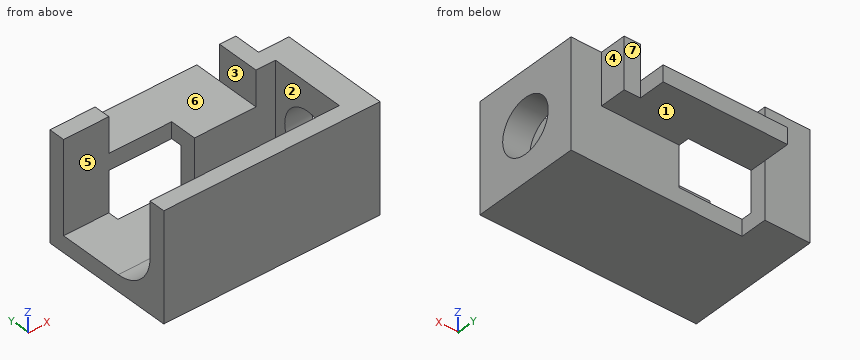
from build123d import *

# Parameters (mm, degrees)
F0_W      = 40
F0_H      = 20
F1_DEPTH  = 10
F3_W      = 35
F3_H      = 3
F4_DEPTH  = 10
F5_W      = 23
F5_H      = 3
F6_DEPTH  = 6.5
F7_W      = 23
F7_H      = 3
F8_DEPTH  = 5
F9_DEPTH  = 10
F10_DEPTH = 35
F11_DEPTH = 40
F12_DEPTH = 35
F13_DEPTH = 40
F14_DEPTH = 35
F15_W     = 20
F15_H     = 17
F16_DEPTH = 5


with BuildPart() as f1:
    # F0 (on Top) → F1 (new body)
    with BuildSketch(Plane.XY):
        Rectangle(F0_W, F0_H)
    extrude(amount=F1_DEPTH)

    # F3 (on face) → F4 (join)
    with BuildSketch(Plane.XY.offset(10)):
        Polygon((20, -10), (20, 10), (15, 10), (15, 7), (15, -7), (15, -10), align=None)
        with Locations((-2.5, 8.5)):
            Rectangle(F3_W, F3_H)
        with Locations((-2.5, -8.5)):
            Rectangle(F3_W, F3_H)
    extrude(amount=F4_DEPTH)

    # F5 (on face) → F6 (cut)
    with BuildSketch(Plane.XY.offset(20)):
        with Locations((-0.1296941414, 8.5)):
            Rectangle(F5_W, F5_H)
    extrude(amount=-F6_DEPTH, mode=Mode.SUBTRACT)

    # F7 (on face) → F8 (join)
    with BuildSketch(Plane(origin=(0, 10, 0), x_dir=(-1, 0, 0), z_dir=(0, 1, 0))):
        with Locations((0.1296941414, 12)):
            Rectangle(F7_W, F7_H)
        Polygon((-11.3703058586, 10.5), (-11.3703058586, 13.5), (-11.3703058586, 20), (-14.3703058586, 20), (-14.3703058586, 10.5), align=None)
        Polygon((11.6296941414, 20), (11.6296941414, 13.5), (11.6296941414, 10.5), (11.6296941414, 0), (20, 0), (20, 20), align=None)
    extrude(amount=F8_DEPTH)

    # F7 (on face) → F9 (join)
    with BuildSketch(Plane(origin=(0, 10, 0), x_dir=(-1, 0, 0), z_dir=(0, 1, 0))):
        with Locations((0.1296941414, 12)):
            Rectangle(F7_W, F7_H)
    extrude(amount=F9_DEPTH)

    # F2 (on face) → F10 (cut)
    with BuildSketch(Plane(origin=(-20, 0, 0), x_dir=(0, -1, 0), z_dir=(-1, 0, 0))):
        with BuildLine():
            Line((-5, 10), (-7, 10))
            ThreePointArc((-7, 10), (-4.9497474683, 5.0502525317), (0, 3))
            Line((0, 3), (0, 5))
            ThreePointArc((0, 5), (-3.5355339059, 6.4644660941), (-5, 10))
        make_face()
        with BuildLine():
            ThreePointArc((0, 5), (3.5355339059, 6.4644660941), (5, 10))
            Line((5, 10), (0, 10))
            Line((0, 10), (0, 5))
        make_face()
    extrude(amount=-F10_DEPTH, mode=Mode.SUBTRACT)

    # F2 (on face) → F11 (cut)
    with BuildSketch(Plane(origin=(-20, 0, 0), x_dir=(0, -1, 0), z_dir=(-1, 0, 0))):
        with BuildLine():
            Line((0, 10), (5, 10))
            ThreePointArc((5, 10), (0, 15), (-5, 10))
            Line((-5, 10), (0, 10))
        make_face()
        with BuildLine():
            ThreePointArc((0, 5), (3.5355339059, 6.4644660941), (5, 10))
            Line((5, 10), (0, 10))
            Line((0, 10), (0, 5))
        make_face()
        with BuildLine():
            Line((0, 10), (-5, 10))
            ThreePointArc((-5, 10), (-3.5355339059, 6.4644660941), (0, 5))
            Line((0, 5), (0, 10))
        make_face()
    extrude(amount=-F11_DEPTH, mode=Mode.SUBTRACT)

    # F2 (on face) → F12 (cut)
    with BuildSketch(Plane(origin=(-20, 0, 0), x_dir=(0, -1, 0), z_dir=(-1, 0, 0))):
        with BuildLine():
            Line((0, 10), (-5, 10))
            ThreePointArc((-5, 10), (-3.5355339059, 6.4644660941), (0, 5))
            Line((0, 5), (0, 10))
        make_face()
        with BuildLine():
            Line((-5, 10), (-7, 10))
            ThreePointArc((-7, 10), (-4.9497474683, 5.0502525317), (0, 3))
            Line((0, 3), (0, 5))
            ThreePointArc((0, 5), (-3.5355339059, 6.4644660941), (-5, 10))
        make_face()
        with BuildLine():
            ThreePointArc((0, 3), (-4.9497474683, 5.0502525317), (-7, 10))
            Line((-7, 10), (-7, 3))
            Line((-7, 3), (0, 3))
        make_face()
    extrude(amount=-F12_DEPTH, mode=Mode.SUBTRACT)

    # F2 (on face) → F13 (cut)
    with BuildSketch(Plane(origin=(-20, 0, 0), x_dir=(0, -1, 0), z_dir=(-1, 0, 0))):
        with BuildLine():
            Line((0, 10), (-5, 10))
            ThreePointArc((-5, 10), (-3.5355339059, 6.4644660941), (0, 5))
            Line((0, 5), (0, 10))
        make_face()
    extrude(amount=-F13_DEPTH, mode=Mode.SUBTRACT)

    # F2 (on face) → F14 (cut)
    with BuildSketch(Plane(origin=(-20, 0, 0), x_dir=(0, -1, 0), z_dir=(-1, 0, 0))):
        with BuildLine():
            ThreePointArc((0, 3), (4.9497474683, 5.0502525317), (7, 10))
            Line((7, 10), (5, 10))
            ThreePointArc((5, 10), (3.5355339059, 6.4644660941), (0, 5))
            Line((0, 5), (0, 3))
        make_face()
    extrude(amount=-F14_DEPTH, mode=Mode.SUBTRACT)

    # F15 (on face) → F16 (cut)
    with BuildSketch(Plane.XZ.offset(-7)):
        with Locations((-10, 11.5)):
            Rectangle(F15_W, F15_H)
    extrude(amount=-F16_DEPTH, mode=Mode.SUBTRACT)


solid = f1.part
The model under review builds one solid part; all positions refer to its coordinate system, in mm. Face numbers are marked on the shaded views. A direction names the side the tool comes from. Round coordinates to 2 decimals unless told otherwise and drop trailing zeros. Order: outer loops, then holes, each group sorted by start corner. A loop starts at its lowest first (then second) coordinate and runs counter-clockwise, first axis right, second up. Notation, with made-up numbers: (-16.5, 7.25) -> (23.5, 7.25) arc R23 cw to (23.5, 44.25) -> close; hole circle Ø5 at (65, 27.25). An arc over 180 degrees is marked (long way). Write item = value, one per line. Start each with the question number.
Item 1: Clearance check with flat-ended pins moving along their axes: pin 1 Ø9.5 at (x, y) = (5, 9) entering from +Z; pin 2 Ø2 at (y, z) = (0.5, 15.5) entering from -X; pin 3 Ø4 at (x, y) = (-4.5, -4) entering from +Z. State where each tip first meets the part, or that it passes through.
Item 2: For line 1 along Z through (x, y) = (17.2, 0); line 2 along Y through (x, z) = (16.9, 10); line 3 along Y through (x, z) = (7, 12.75), list the stretches that pass through material, from the lowest coordinate up.
Item 3: Consider section D-D on z = 1. Write out the cut boundary in (x, y), plus the area to 3 significant figures.
Item 4: Consider section B-B on z = 14.5. Write out the cut boundary in (x, y), plus the area to 3 significant figures.
Item 5: Consider section A-A on y = 10.75. Write out the cut boundary in (x, z), plus the area to 3 significant figures.
Item 6: Mouldability with a two-part tool opening along X and no side actions: class the marked faces 1, 2, 3 and 4 as released by +X, released by -X, zero draft, split by the parting line, or undercut.
Item 7: For the marked faces 5, 6 and 7, list the 3-axis set-ups (+Z, -Z, +X, -X, +Y, -Y) from which the entire face can be reached by the end or side of a thin tool; tool diameter is ignored.
Item 8: Consider section C-C on x = -15. Write out the cut boundary in (y, z).
Conclusion:
q1.pin_1 = 13.5
q1.pin_2 = 15
q1.pin_3 = 6.39
q2.line_1 = 0 to 5, 15 to 20
q2.line_2 = -10 to -5, 5 to 10
q2.line_3 = -10 to -7, 7 to 20
q3.outline = (-20, -10) -> (20, -10) -> (20, 10) -> (-11.63, 10) -> (-11.63, 15) -> (-20, 15) -> close
q3.area = 842 mm2
q4.outline = (-20, -10) -> (20, -10) -> (20, -2.18) -> (15, -2.18) -> (15, -7) -> (-20, -7) -> close; (-20, 12) -> (-11.63, 12) -> (-11.63, 15) -> (-20, 15) -> close; (11.37, 7) -> (15, 7) -> (15, 2.18) -> (20, 2.18) -> (20, 10) -> (14.37, 10) -> (14.37, 15) -> (11.37, 15) -> close
q4.area = 234 mm2
q5.outline = (-20, 0) -> (-11.63, 0) -> (-11.63, 3) -> (-20, 3) -> close; (0, 10.5) -> (14.37, 10.5) -> (14.37, 20) -> (11.37, 20) -> (11.37, 13.5) -> (0, 13.5) -> close
q5.area = 87.7 mm2
q6.face_1 = zero draft
q6.face_2 = released by -X
q6.face_3 = undercut
q6.face_4 = released by +X
q7.face_5 = +Z, -X
q7.face_6 = +Z, +Y
q7.face_7 = +Z, -Z, +X, +Y
q8.outline = (-10, 0) -> (15, 0) -> (15, 20) -> (12, 20) -> (12, 3) -> (0, 3) arc R7 cw to (-7, 10) -> (-7, 20) -> (-10, 20) -> close
